from build123d import *

# Parameters (mm, degrees)
F0_W      = 100
F0_H      = 60
F1_DEPTH  = 30
F2_R      = 10.1
F3_DEPTH  = 25
F4_R      = 5.1
F5_DEPTH  = 30.001
F9_R      = 2.5
F10_DEPTH = 10
F11_R     = 2.5
F12_DEPTH = 10
F13_R     = 2.5
F14_DEPTH = 10


with BuildPart() as f1:
    # F0 (on Top) → F1 (new body)
    with BuildSketch(Plane.XY):
        Rectangle(F0_W, F0_H)
    extrude(amount=F1_DEPTH)

    # F2 (on face) → F3 (cut)
    with BuildSketch(Plane.XY.offset(30)):
        Circle(F2_R)
    extrude(amount=-F3_DEPTH, mode=Mode.SUBTRACT)

    # F4 (on face) → F5 (cut, through all)
    with BuildSketch(Plane.XY.offset(30)):
        with Locations((-40, 20)):
            Circle(F4_R)
        with Locations((-40, -20)):
            Circle(F4_R)
        with Locations((40, 20)):
            Circle(F4_R)
        with Locations((40, -20)):
            Circle(F4_R)
    extrude(amount=-F5_DEPTH, mode=Mode.SUBTRACT)

    # F6 (on Right) → F8 (revolve, cut)
    with BuildSketch(Plane.YZ):
        Polygon((0, 10.5), (0, 0), (10.5, 0), align=None)
    revolve(axis=Axis((0, 0, -23.476606), (0, 0, -1)), mode=Mode.SUBTRACT)

    # F9 (on face) → F10 (cut)
    with BuildSketch(Plane.XZ.offset(30)):
        with Locations((-40, 15)):
            Circle(F9_R)
        with Locations((40, 15)):
            Circle(F9_R)
    extrude(amount=-F10_DEPTH, mode=Mode.SUBTRACT)

    # F11 (on face) → F12 (cut)
    with BuildSketch(Plane(origin=(0, 30, 0), x_dir=(-1, 0, 0), z_dir=(0, 1, 0))):
        with Locations((-40, 15)):
            Circle(F11_R)
        with Locations((40, 15)):
            Circle(F11_R)
    extrude(amount=-F12_DEPTH, mode=Mode.SUBTRACT)

    # F13 (on face) → F14 (cut)
    with BuildSketch(Plane.XY.offset(30)):
        with Locations((0, 13.5)):
            Circle(F13_R)
    extrude(amount=-F14_DEPTH, mode=Mode.SUBTRACT)


solid = f1.part
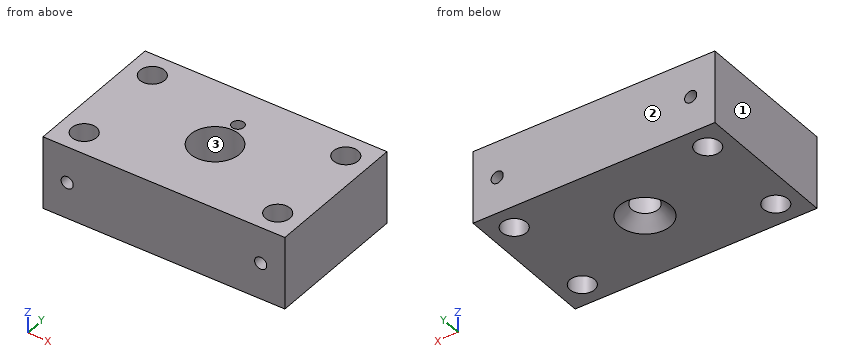
For this review, take the finished solid that the model builds, in its own axes (mm). Face numbers are marked on the shaded views. Give positions to 0.01 mm unless a question says otherwise; leave off trailing zeros. Order: outer loops, then holes, each group sorted by start corner. A loop starts at its lowest first (then second) coordinate and runs counter-clockwise, first axis right, second up. Notation, with made-up numbers: (26, 39.5) - (42, 39.5) arc R17 ccw to (42, 54.5) - close; hole circle Ø11 at (-21.75, 75.5). An arc over 180 degrees is marked (long way). Answer as a JSON object with one key per item and string values. Group by question number.
Item 1: Take a section at A-A on x = 40. Give the boundary of the cut face in (y, z).
Item 2: Wall thickness on line 1 along X through (y, z) = (-27.3, 15); line 2 along Y through (x, z) = (0, 22); line 3 along Y through (x, z) = (37, 10): over which ranges is each line inside the solid? List them lowest first.
Item 3: Take a section at B-B on z = 15. Give the boundary of the cut face in (x, y), and give its area (3 significant figures).
Item 4: Take a section at C-C on y = -20. Give the boundary of the cut face in (x, z).
Item 5: Draft analysis for pull direction Y (two halves, no side actions). For the marked faces 1, 2 and 3, state which applies: pulls with the +Y half, pulls with the -Y half, needs draft (parallel to the pull), parting line crosses it, or undercut.
Item 6: Take a section at D-D on x = 0. Give the boundary of the cut face in (y, z), and give its area (4 significant figures).
Item 7: Clearance check with flat-ended pins moving along their axes: pin 1 Ø1 at (x, y) = (-39.5, -23.5) entering from +Z; pin 2 Ø2.5 at (x, y) = (0, 13) entering from +Z; pin 3 Ø18 at (x, y) = (0, 0) entering from -Z. State where each tip first meets the part, or that it passes through.
Reported:
{
 "1": {"outline": "(-30, 0) - (-25.1, 0) - (-25.1, 12.5) - (-30, 12.5) - close; (-30, 17.5) - (-25.1, 17.5) - (-25.1, 30) - (-30, 30) - close; (-14.9, 0) - (14.9, 0) - (14.9, 30) - (-14.9, 30) - close; (25.1, 0) - (30, 0) - (30, 12.5) - (25.1, 12.5) - close; (25.1, 17.5) - (30, 17.5) - (30, 30) - (25.1, 30) - close"},
 "2": {"line 1": "-50 to -42.5, -37.5 to 37.5, 42.5 to 50", "line 2": "-30 to -10.1, 10.1 to 11, 16 to 30", "line 3": "-30 to -24.12, -15.88 to 15.88, 24.12 to 30"},
 "3": {"outline": "(-50, -30) - (-42.5, -30) - (-42.5, -24.45) arc R5.1 cw (long way) to (-37.5, -24.45) - (-37.5, -30) - (37.5, -30) - (37.5, -24.45) arc R5.1 cw (long way) to (42.5, -24.45) - (42.5, -30) - (50, -30) - (50, 30) - (42.5, 30) - (42.5, 24.45) arc R5.1 cw (long way) to (37.5, 24.45) - (37.5, 30) - (-37.5, 30) - (-37.5, 24.45) arc R5.1 cw (long way) to (-42.5, 24.45) - (-42.5, 30) - (-50, 30) - close; hole circle Ø20.2 at (0, 0)", "area": "5,250 mm^2"},
 "4": {"outline": "(-50, 0) - (-45.1, 0) - (-45.1, 30) - (-50, 30) - close; (-34.9, 0) - (34.9, 0) - (34.9, 30) - (-34.9, 30) - close; (45.1, 0) - (50, 0) - (50, 30) - (45.1, 30) - close"},
 "5": {"face 1": "needs draft", "face 2": "pulls with the +Y half", "face 3": "undercut"},
 "6": {"outline": "(-30, 0) - (-10.5, 0) - (-5.5, 5) - (-10.1, 5) - (-10.1, 30) - (-30, 30) - close; (5.5, 5) - (10.5, 0) - (30, 0) - (30, 30) - (16, 30) - (16, 20) - (11, 20) - (11, 30) - (10.1, 30) - (10.1, 5) - close", "area": "1,165 mm^2"},
 "7": {"pin 1": "through", "pin 2": "z = 20", "pin 3": "z = 1.5"}
}
